Here's how the part is built. I have some questions about the finished solid (model axes, mm). A direction names the side the tool comes from. Coordinates: 2 decimals unless noted, no trailing zeros. Loops run counter-clockwise (first coordinate to the right, second up) from the corner with the lowest first, then second, coordinate; pieces in that order, holes last.
from build123d import *

# Parameters (mm, degrees)
SKETCH1_W                    = 387.4
SKETCH1_H                    = 106
BASE_FLANGE1_DEPTH           = 2
EDGE_FLANGE1_STRIP_W         = 9.4732
EDGE_FLANGE1_STRIP_H         = 2
EDGE_FLANGE1_STRIP_CUT_DEPTH = 387.4
EDGE_FLANGE1_DEPTH           = 387.4
EDGE_FLANGE2_STRIP_W         = 9.4732
EDGE_FLANGE2_STRIP_H         = 2
EDGE_FLANGE2_STRIP_CUT_DEPTH = 387.4
EDGE_FLANGE2_DEPTH           = 387.4
SKETCH14_W                   = 73.905952632
SKETCH14_H                   = 44.03163087
CUT_EXTRUDE1_DEPTH           = 4
MIRROR2_COPY_1_SKETCH_W      = 73.905952632
MIRROR2_COPY_1_SKETCH_H      = 44.03163087
MIRROR2_COPY_1_DEPTH         = 4
CUT_EXTRUDE2_DEPTH           = 221.95178207
CUT_EXTRUDE2_DEPTH_BACK      = 221.95178207
SKETCH15_R                   = 2.5


# Sheet-metal steps are written as plain solids
with BuildPart() as part:
    # Sketch1 → Base-Flange1 (new body)
    with BuildSketch(Plane.XY):
        Rectangle(SKETCH1_W, SKETCH1_H)
    extrude(amount=-BASE_FLANGE1_DEPTH)

    # Edge-Flange1 strip (across the edge) → Edge-Flange1 strip cut (cut)
    with BuildSketch(Plane(origin=(193.7, 53, 0), x_dir=(0, -1, 0), z_dir=(-1, 0, 0))):
        with Locations((-2, -1)):
            Rectangle(EDGE_FLANGE1_STRIP_W, EDGE_FLANGE1_STRIP_H)
    extrude(amount=EDGE_FLANGE1_STRIP_CUT_DEPTH, mode=Mode.SUBTRACT)

    # Edge-Flange1 section (across the edge) → Edge-Flange1 (add)
    with BuildSketch(Plane(origin=(193.7, 53, 0), x_dir=(0, -1, 0), z_dir=(-1, 0, 0))):
        with BuildLine():
            Line((0, 0.7366), (0, 8))
            Line((0, 8), (2, 8))
            Line((2, 8), (2, 0.7366))
            ThreePointArc((2, 0.7366), (2.215745145, 0.215745145), (2.7366, 0))
            Line((2.7366, 0), (2.7366, -2))
            ThreePointArc((2.7366, -2), (0.801531583, -1.198468417), (0, 0.7366))
        make_face()
    extrude(amount=EDGE_FLANGE1_DEPTH)

    # Edge-Flange2 strip (across the edge) → Edge-Flange2 strip cut (cut)
    with BuildSketch(Plane(origin=(-193.7, -53, 0), x_dir=(0, 1, 0), z_dir=(1, 0, 0))):
        with Locations((-2, -1)):
            Rectangle(EDGE_FLANGE2_STRIP_W, EDGE_FLANGE2_STRIP_H)
    extrude(amount=EDGE_FLANGE2_STRIP_CUT_DEPTH, mode=Mode.SUBTRACT)

    # Edge-Flange2 section (across the edge) → Edge-Flange2 (add)
    with BuildSketch(Plane(origin=(-193.7, -53, 0), x_dir=(0, 1, 0), z_dir=(1, 0, 0))):
        with BuildLine():
            Line((0, 0.7366), (0, 8))
            Line((0, 8), (2, 8))
            Line((2, 8), (2, 0.7366))
            ThreePointArc((2, 0.7366), (2.215745145, 0.215745145), (2.7366, 0))
            Line((2.7366, 0), (2.7366, -2))
            ThreePointArc((2.7366, -2), (0.801531583, -1.198468417), (0, 0.7366))
        make_face()
    extrude(amount=EDGE_FLANGE2_DEPTH)

    # Sketch14 → Cut-Extrude1 (cut)
    with BuildSketch(Plane(origin=(0, 53, 0), x_dir=(1, 0, 0), z_dir=(0, 1, 0))):
        with Locations((-218.652976316, 2.389975087)):
            Rectangle(SKETCH14_W, SKETCH14_H)
    cut_extrude1 = extrude(amount=-CUT_EXTRUDE1_DEPTH, mode=Mode.SUBTRACT)

    # Mirror1: Cut-Extrude1 across plane
    add(cut_extrude1.mirror(Plane.ZX), mode=Mode.SUBTRACT)

    # Mirror2: Cut-Extrude1 across plane
    add(cut_extrude1.mirror(Plane(origin=(0, 0, 0), x_dir=(0, 0, 1), z_dir=(1, 0, 0))), mode=Mode.SUBTRACT)

    # Mirror2 copy 1 sketch → Mirror2 copy 1 (cut)
    with BuildSketch(Plane(origin=(0, -53, 0), x_dir=(-1, 0, 0), z_dir=(0, -1, 0))):
        with Locations((-218.652976316, 2.389975087)):
            Rectangle(MIRROR2_COPY_1_SKETCH_W, MIRROR2_COPY_1_SKETCH_H)
    extrude(amount=-MIRROR2_COPY_1_DEPTH, mode=Mode.SUBTRACT)

    # Sketch15 → Cut-Extrude2 (cut, two sides: drawn at the far end of the back side and taken through both)
    with BuildSketch(Plane(origin=(0, 53, 0), x_dir=(1, 0, 0), z_dir=(0, 1, 0)).offset(-CUT_EXTRUDE2_DEPTH_BACK)):
        with Locations(Location((151.7, -4.5, 0), (0, 0, 270))):
            Circle(SKETCH15_R)
        with Locations(Location((0, -4.5, 0), (0, 0, 270))):
            Circle(SKETCH15_R)
        with Locations(Location((-151.7, -4.5, 0), (0, 0, 270))):
            Circle(SKETCH15_R)
    extrude(amount=CUT_EXTRUDE2_DEPTH + CUT_EXTRUDE2_DEPTH_BACK, mode=Mode.SUBTRACT)


solid = part.part
Q1. Will these pins go through, and if not, where does the flat tip stop? P1, Ø5, axis at x = -1, y = 33.5, coming from the +Z side; P2, Ø3, axis at x = -151.7, z = 4.5, coming from the -Y side; P3, Ø4.5, axis at y = 51.5, z = 2.5, coming from the +X side; P4, Ø1.6, axis at x = -188, z = -1, coming from the +Y side.
Q2. For faces 4 (the flat face through (3, 53, 4)), 5 (the flat face through (-3, -51, 4)), which set-ups out of +Z, -Z, +X, -X, +Y, -Y let a thin tool reach every point of the face, with its end or its side?
Q3. We'd pull the mould along Y, two halves only. Please class faces 1 (the flat face through (-3, -53, 4)), 2 (the flat face through (-3, 1, -2)), 3 (the flat face through (-3, 1, 0)): pulls with the +Y half, pulls with the -Y half, needs draft (parallel to the pull), parting line crosses it, or undercut.
Q4. Suppose I cut it at C-C on y = 27.5. Write out the boundary of the cut face in (x, z).
Q5. Suppose I cut it at B-B on x = 31. Write out the boundary of the cut face in (y, z).
Q6. Please list where these lines run through material, in increasing order: probe 1 along X at (y, z) = (52.45, 4.5); probe 2 along Y at (x, z) = (130, 7.25); probe 3 along Y at (x, z) = (-142, 0.25).
Q7. Suppose I cut it at A-A on z = 4.5. State how many separate pieces and enclosed holes the cut face has, and give its area (3 significant figures).
Check values:
1. P1: stops at z = 0
1. P2: passes through
1. P3: stops at x = 181.7
1. P4: stops at y = 49
2. face 4: +Z, -Z, +X, -X, +Y
2. face 5: +Z, +X, -X
3. face 1: pulls with the -Y half
3. face 2: needs draft
3. face 3: undercut
4. outline: (-193.7, -2) - (193.7, -2) - (193.7, 0) - (-193.7, 0) - close
5. outline: (-53, 0.74) arc R2.74 ccw to (-50.26, -2) - (50.26, -2) arc R2.74 ccw to (53, 0.74) - (53, 8) - (51, 8) - (51, 0.74) arc R0.74 cw to (50.26, 0) - (-50.26, 0) arc R0.74 cw to (-51, 0.74) - (-51, 8) - (-53, 8) - close
6. probe 1: x = -181.7 to -154.2, -149.2 to -2.5, 2.5 to 149.2, 154.2 to 181.7
6. probe 2: y = -53 to -51, 51 to 53
6. probe 3: y = -52.96 to -50.82, 50.82 to 52.96
7. separate pieces: 8
7. enclosed holes: 0
7. area: 1,390 mm2
